For this review, use the dimensioned drawing (mm, ordinates from the lowest corner) and the shaded views. Give positions to 0.01 mm unless a question says otherwise; leave off trailing zeros. Order: outer loops, then holes, each group sorted by start corner. A loop starts at its lowest first (then second) coordinate and runs counter-clockwise, first axis right, second up. Notation, with made-up numbers: (75, 9) - (80, 9) arc R31 ccw to (80, 39) - close; hole circle Ø10 at (59.5, 10). An arc over 180 degrees is marked (long way). One line per item, written item: value.
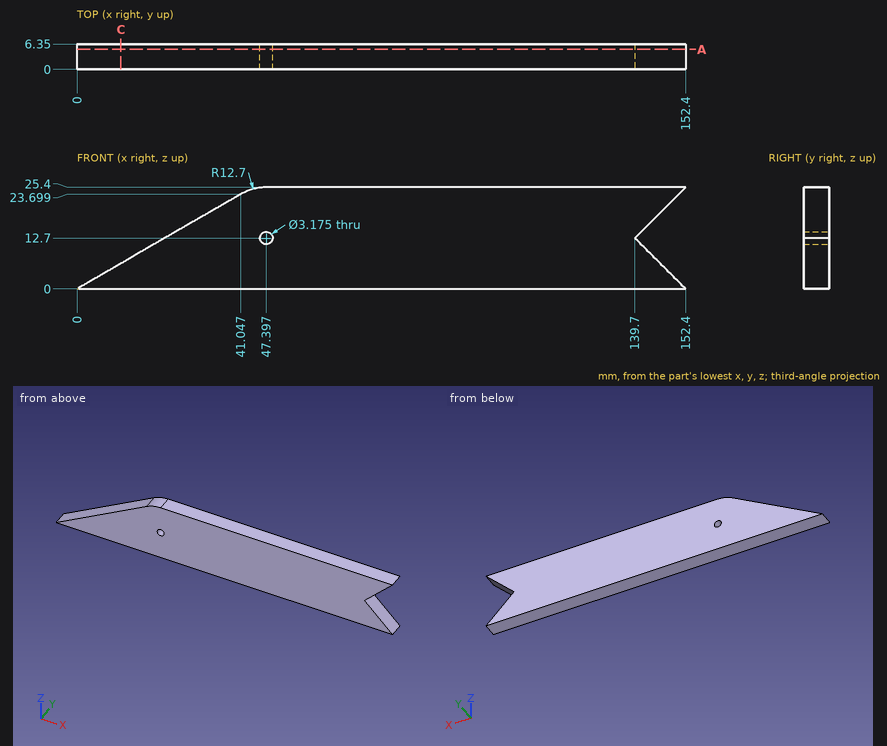
(1) Wall thickness on line 1 (X direction, y = 3, z = 12.7) (1 decimal); line 2 (Z direction, x = 143, y = 4.25); line 3 (X direction, y = 2.5, z = 13.5) (1 decimal): over which ranges is each line inside the solid? List them lowest first. Write a range as from..to.
Answers below:
line 1: x = 22..45.8, 49..139.7
line 2: z = 0..9.4, 16..25.4
line 3: x = 23.4..46, 48.8..140.5
(2) Take a section at A-A (y = 5). Write out the cut boundary in (x, z) (1 decimal), then the cut area to 3 significant figures.
Answers below:
outline: (0, 0) - (152.4, 0) - (139.7, 12.7) - (152.4, 25.4) - (47.4, 25.4) arc R12.7 ccw to (41, 23.7) - close; hole circle Ø3.2 at (47.4, 12.7)
area: 3,140 mm^2
(3) Take a section at C-C (x = 11). Write out the cut boundary in (y, z).
Answers below:
outline: (0, 0) - (6.35, 0) - (6.35, 6.35) - (0, 6.35) - close
(4) For P1, Ø3, axis at y = 2.5, z = 14.5, coming from the +X side, flat-tipped, find the tip position at first contact; note if it passes through.
Answers below:
P1: stops at x = 143
